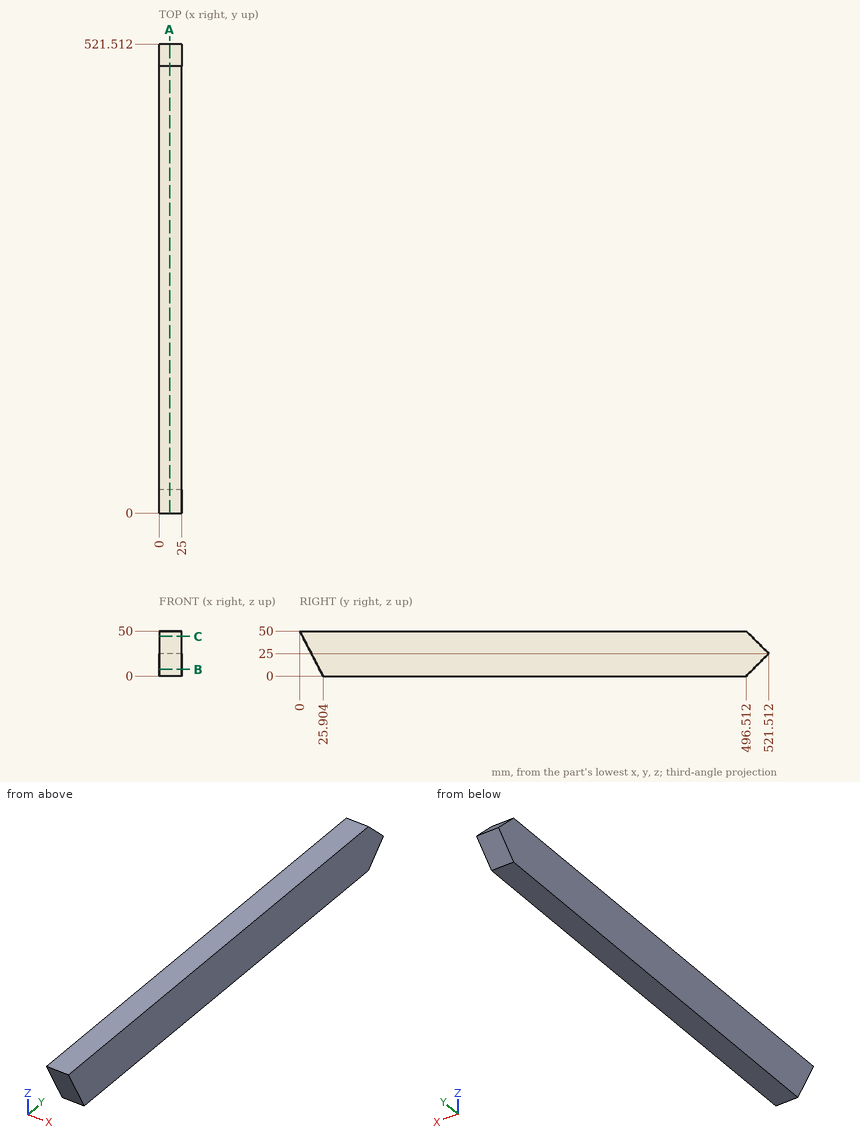
For this review, use the dimensioned drawing (mm, ordinates from the lowest corner) and the shaded views. Coordinates: 2 decimals unless noted, no trailing zeros. Write each loop counter-clockwise with the first axis right and the second up, starting at its lowest first coordinate (ties: lowest second). Pieces come first, ordered by that corner, then holes. Notation, with made-up numbers: (32, 31) -> (82, 31) arc R17 ccw to (82, 57) -> close; hole circle Ø11 at (55, 63.5). An arc over 180 degrees is marked (long way). Write each question's results on one line, items separated by ' | '. Start each with the question number.
(1) Take a section at B-B on z = 7.5. Write out the cut boundary in (x, y), and give its area (4 significant figures).
(2) Clearance check with flat-ended pins moving along their axes: P1, Ø4, axis at x = 14, z = 5.5, coming from the -Y side; P2, Ø10, axis at x = 13, z = 29, coming from the -Y side; P3, Ø1.5, axis at x = 19.5, z = 42.5, coming from the -Y side. State where each tip first meets the part, or that it passes through.
(3) Take a section at C-C on z = 44. Write out the cut boundary in (x, y), and give its area (3 significant figures).
(4) For line 1 along Y through (x, z) = (19.5, 6.5) (1 decimal); line 2 along Y through (x, z) = (23.5, 10.5) (1 decimal), list the stretches that pass through material, from the lowest coordinate up. Write a range as from..to.
(5) Take a section at A-A on x = 11.5. Write out the cut boundary in (y, z).
Results found:
1) outline: (0, 22.02) -> (25, 22.02) -> (25, 504.01) -> (0, 504.01) -> close | area: 12,050 mm2
2) P1: stops at y = 22.02 | P2: stops at y = 8.29 | P3: stops at y = 3.5
3) outline: (0, 3.11) -> (25, 3.11) -> (25, 502.51) -> (0, 502.51) -> close | area: 12,500 mm2
4) line 1: y = 22.5..503 | line 2: y = 20.5..507
5) outline: (0, 50) -> (25.9, 0) -> (496.51, 0) -> (521.51, 25) -> (496.51, 50) -> close
